CAD build for the part. Positions are in the model's coordinates, mm. Round coordinates to 2 decimals unless told otherwise and drop trailing zeros. Write each loop counter-clockwise with the first axis right and the second up, starting at its lowest first coordinate (ties: lowest second). Pieces come first, ordered by that corner, then holes. Notation, with made-up numbers: (-22.5, -26.5) -> (5.5, -26.5) arc R4 ccw to (5.5, -21.5) -> close; hole circle Ø2 at (-5.75, 32). An arc over 180 degrees is marked (long way). Put each result on its own line as item: value. Start each with the question number.
1. Drill centre lines: line 1 (Y direction, x = 105, z = 1); line 2 (Y direction, x = 3.2, z = 1); line 3 (X direction, y = -11.5, z = 0.5). Where is each one in solid material? Low to high. Write a range as from..to.
2. Saw through at D-D on z = 0.7. State how many separate pieces and enclosed holes the cut face has, and give its area (3 significant figures).
3. Saw through at A-A on x = 3.2. List the corners of the cut face in (y, z), and give its area (3 significant figures).
4. Saw through at C-C on x = 105. List the corners of the cut face in (y, z).
5. Saw through at B-B on y = -12.7. List the corners of the cut face in (x, z), and give its area (3 significant figures).
6. Pull direction Y, two halves, no side cores. Call faces 1 (the cylindrical face through (2.875, -14.164, 1.479)), 2 (the flat face through (54, -25.4, 1)), 3 (the flat face through (54, -13, 0)): pulls with the +Y half, pulls with the -Y half, needs draft (parallel to the pull), parting line crosses it, or undercut.
7. Flat gauge pins, fed straight in: P1, Ø5, axis at x = 3.2, y = -12.7, coming from the -Z side; P2, Ø2.5, axis at x = 17.45, y = -20.93, coming from the -Z side. Where does each tip first touch, or does it go through?
from build123d import *

# Parameters (mm, degrees)
SKETCH1_W           = 110
SKETCH1_H           = 25.4
SKETCH1_R           = 1.5
SKETCH1_R_2         = 4
BOSS_EXTRUDE1_DEPTH = 3


with BuildPart() as part:
    # Sketch1 → Boss-Extrude1 (new body)
    with BuildSketch(Plane.XY):
        with Locations((55, -12.7)):
            Rectangle(SKETCH1_W, SKETCH1_H)
        with Locations((3.2, -12.7)):
            Circle(SKETCH1_R, mode=Mode.SUBTRACT)
        with Locations((7.95, -4.472758664)):
            Circle(SKETCH1_R, mode=Mode.SUBTRACT)
        with Locations((17.45, -4.472758664)):
            Circle(SKETCH1_R, mode=Mode.SUBTRACT)
        with Locations((22.2, -12.7)):
            Circle(SKETCH1_R, mode=Mode.SUBTRACT)
        with Locations((17.45, -20.927241336)):
            Circle(SKETCH1_R, mode=Mode.SUBTRACT)
        with Locations((7.95, -20.927241336)):
            Circle(SKETCH1_R, mode=Mode.SUBTRACT)
        with Locations((12.7, -12.7)):
            Circle(SKETCH1_R_2, mode=Mode.SUBTRACT)
        with Locations(Location((105, -4.472758664, 0), (0, 0, 180))):
            Circle(SKETCH1_R, mode=Mode.SUBTRACT)
        with Locations((105, -20.927241336)):
            Circle(SKETCH1_R, mode=Mode.SUBTRACT)
    extrude(amount=BOSS_EXTRUDE1_DEPTH)


solid = part.part
Return value:
1. line 1: y = -25.4..-22.43, -19.43..-5.97, -2.97..0
1. line 2: y = -25.4..-14.2, -11.2..0
1. line 3: x = 0..2.3, 4.1..8.88, 16.52..21.3, 23.1..110
2. separate pieces: 1
2. enclosed holes: 9
2. area: 2,690 mm^2
3. outline: (-25.4, 0) -> (-14.2, 0) -> (-14.2, 3) -> (-25.4, 3) -> close; (-11.2, 0) -> (0, 0) -> (0, 3) -> (-11.2, 3) -> close
3. area: 67.2 mm^2
4. outline: (-25.4, 0) -> (-22.43, 0) -> (-22.43, 3) -> (-25.4, 3) -> close; (-19.43, 0) -> (-5.97, 0) -> (-5.97, 3) -> (-19.43, 3) -> close; (-2.97, 0) -> (0, 0) -> (0, 3) -> (-2.97, 3) -> close
5. outline: (0, 0) -> (1.7, 0) -> (1.7, 3) -> (0, 3) -> close; (4.7, 0) -> (8.7, 0) -> (8.7, 3) -> (4.7, 3) -> close; (16.7, 0) -> (20.7, 0) -> (20.7, 3) -> (16.7, 3) -> close; (23.7, 0) -> (110, 0) -> (110, 3) -> (23.7, 3) -> close
5. area: 288 mm^2
6. face 1: undercut
6. face 2: pulls with the -Y half
6. face 3: needs draft
7. P1: stops at z = 0
7. P2: passes through
